Design review of the part shown in the three views and the two pictorial views. Dimensions are in mm from the part's minimum x, y and z. A direction names the side the tool comes from. Coordinates: 2 decimals unless noted, no trailing zeros. Loops run counter-clockwise (first coordinate to the right, second up) from the corner with the lowest first, then second, coordinate; pieces in that order, holes last. Notation, with made-up numbers: (62, 64) - (84, 64) arc R14 ccw to (84, 74) - close; hole circle Ø9 at (10.5, -22.5). An arc over 180 degrees is marked (long way). One line per item, written item: value. Start each with the question number.
1. For the marked faces 1, 2 and 3, list the 3-axis set-ups (+Z, -Z, +X, -X, +Y, -Y) from which the entire face can be reached by the end or side of a thin tool; tool diameter is ignored.
2. To check wall thickness, follow line 1 (Y direction, x = 5, z = 4.75); line 2 (Z direction, x = 19, y = 16.5); line 3 (Y direction, x = 20, z = 21.75). State the ranges of each line that lie inside material, in increasing order. Write a range as from..to.
3. Insertion check: pin 1 (5.5 mm diameter, centred on x = 18.5, z = 23, fed in from -Y); pin 2 (9 mm diameter, centred on x = 7, y = 32, fed in from +Z); pin 3 (2 mm diameter, centred on x = 3, y = 24, fed in from +Z). Each pin has a flat end and moves straight along its axis. Give the tip position at first contact, or say it passes through.
4. Take a section at D-D, the plane z = 13.5. State the section outline as (x, y) points.
5. Take a section at A-A, the plane z = 4.75. State the section outline as (x, y) points.
6. Take a section at C-C, the plane y = 5. State the section outline as (x, z) points, and give its area (3 significant figures).
7. Take a section at B-B, the plane x = 9. State the section outline as (y, z) points.
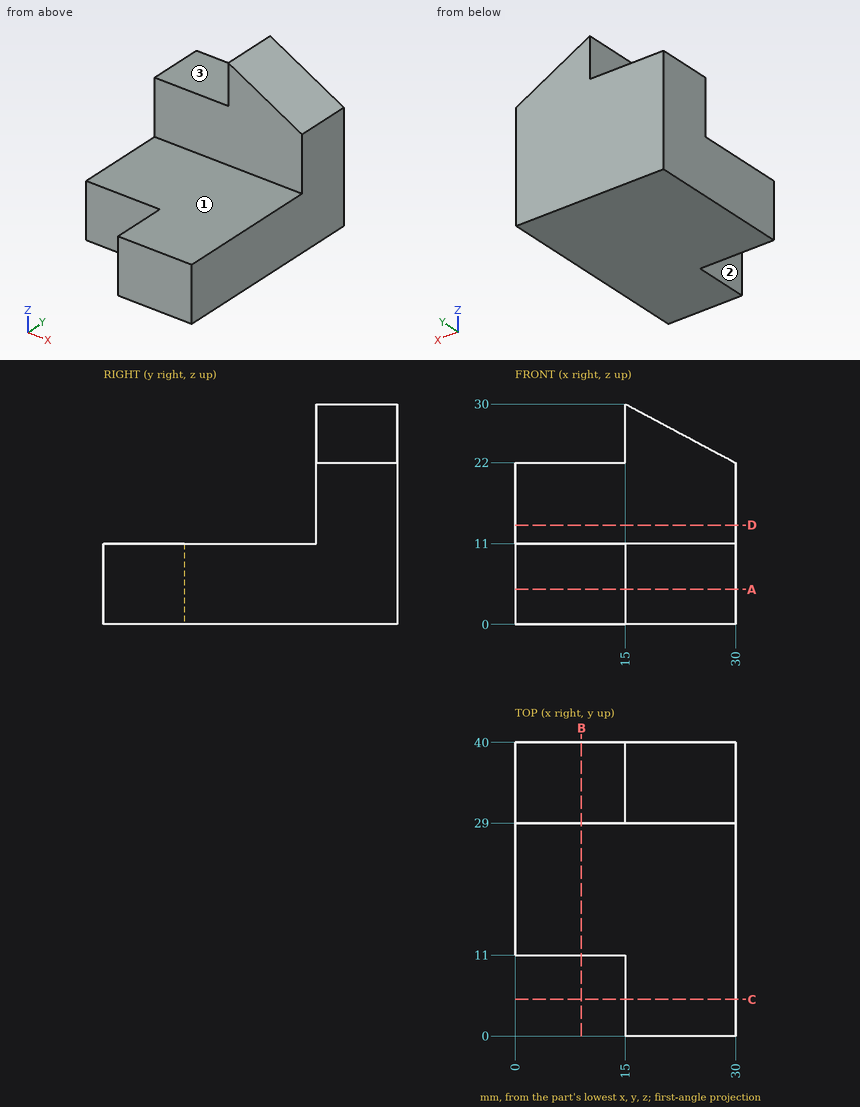
Solutions:
1. face 1: +Z, +X, -X, -Y
1. face 2: +Z, -Z, -X, -Y
1. face 3: +Z, -X, +Y, -Y
2. line 1: 11..40
2. line 2: 0..11
2. line 3: 29..40
3. pin 1: y = 29
3. pin 2: z = 22
3. pin 3: z = 11
4. outline: (0, 29) - (30, 29) - (30, 40) - (0, 40) - close
5. outline: (0, 11) - (15, 11) - (15, 0) - (30, 0) - (30, 40) - (0, 40) - close
6. outline: (15, 0) - (30, 0) - (30, 11) - (15, 11) - close
6. area: 165 mm2
7. outline: (11, 0) - (40, 0) - (40, 22) - (29, 22) - (29, 11) - (11, 11) - close
